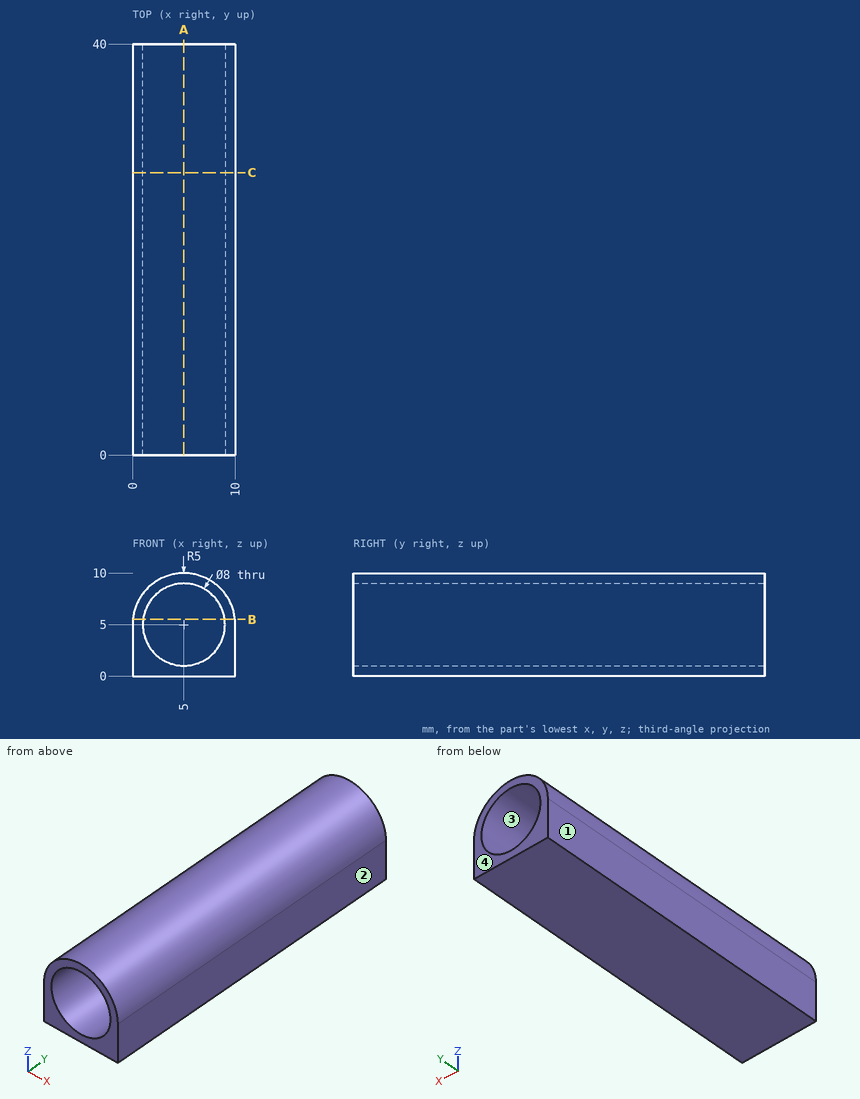
Answer from the drawing. Dimensions are ordinates in mm from the lowest x, y and z of the part. Coordinates: 2 decimals unless noted, no trailing zeros. Write each loop counter-clockwise with the first axis right and the second up, starting at its lowest first coordinate (ties: lowest second). Pieces come first, ordered by that corner, then holes. Notation, with made-up numbers: M 29.5,70.25 L 33.5,70.25 A26 ccw 33.5,98.25 Z; hole C 12.25,58.25 d5. An arc over 180 degrees is marked long. Use a Markdown table: item, result.
Q1. Straight lines are drawn through the part: L1, parallel to Z at x = 5, y = 9; L2, parallel to X at y = 34.5, z = 8.5; L3, parallel to Z at x = 2.25, y = 3. For each, find the intervals that lie inside material, in ascending order. Write a range as [from, to].
Answer block:
| item | result |
|---|---|
| L1 | z = [0, 1], [9, 10] |
| L2 | x = [1.43, 3.06], [6.94, 8.57] |
| L3 | z = [0, 2.1], [7.9, 9.18] |
Q2. Determine the mould class of the marked faces 1, 2, 3 and 4 for opening direction X: released by +X, released by -X, zero draft, split by the parting line, or undercut.
Answer block:
| item | result |
|---|---|
| face 1 | released by -X |
| face 2 | released by +X |
| face 3 | undercut |
| face 4 | zero draft |
Q3. The part is cut by section A-A, the plane x = 5. Write down the section's boundary in (y, z).
Answer block:
| item | result |
|---|---|
| outline | M 0,0 L 40,0 L 40,1 L 0,1 Z; M 0,9 L 40,9 L 40,10 L 0,10 Z |
Q4. The part is cut by section B-B, the plane z = 5.5. Write down the section's boundary in (x, y), then the cut area to 3 significant figures.
Answer block:
| item | result |
|---|---|
| outline | M 0.03,0 L 1.03,0 L 1.03,40 L 0.03,40 Z; M 8.97,0 L 9.97,0 L 9.97,40 L 8.97,40 Z |
| area | 80.5 mm2 |
Q5. Each of these flat-tipped pins is pushed along its axis until it touches: pin 1 Ø2 at (x, z) = (2, 7) entering from -Y; pin 2 Ø1.5 at (x, y) = (2.5, 24) entering from +Z. Where does it stop, or does it pass through?
Answer block:
| item | result |
|---|---|
| pin 1 | stops at y = 0 |
| pin 2 | stops at z = 9.68 |
Q6. The part is cut by section C-C, the plane y = 27.5. Write down the section's boundary in (x, z), then the cut area to 3 significant figures.
Answer block:
| item | result |
|---|---|
| outline | M 0,0 L 10,0 L 10,5 A5 ccw 0,5 Z; hole C 5,5 d8 |
| area | 39.0 mm2 |
